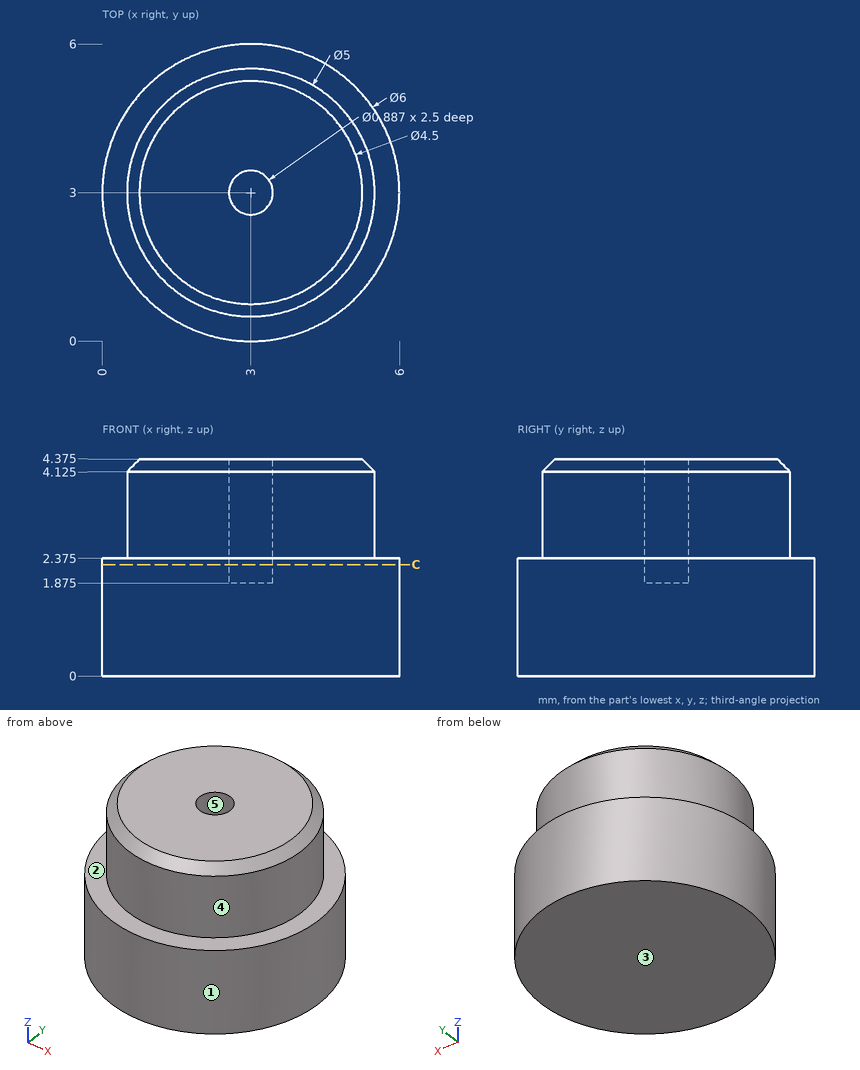
Could you check a few things on this drawing? It's one solid part, dimensions in mm from its lowest x, y, z. A direction names the side the tool comes from. Round coordinates to 2 decimals unless told otherwise and drop trailing zeros. Loops run counter-clockwise (first coordinate to the right, second up) from the corner with the lowest first, then second, coordinate; pieces in that order, holes last.
Q1. On a 3-axis mill with a long thin cutter (end or side, diameter ignored), from which of +Z, -Z, +X, -X, +Y, -Y can I reach the whole of each face in a straight line? I mean the marked faces 1 and 2. Say none if no direction works.
Q2. Thinking about a two-plate mould opening in X: for the marked faces 3, 4 and 5, which applies, pulls with the +X half, pulls with the -X half, needs draft (parallel to the pull), parting line crosses it, or undercut?
Q3. For P1, Ø1.5, axis at y = 2, z = 4, coming from the +X side; P2, Ø1, axis at y = 1, z = 1, coming from the +X side, each with a flat end and sliding along its axis, tell me the tip position at first contact or that it passes through.
Q4. I want a section at C-C (z = 2.25). Write out the boundary of the cut face in (x, y).
Q5. Please list where these lines run through material, in increasing order: L1, parallel to Y at x = 3, z = 3.35; L2, parallel to Z at x = 3.7, y = 5.6 (3 decimals); L3, parallel to Z at x = 5.05, y = 1.85.
Answer below:
1. face 1: +Z, -Z
1. face 2: +Z
2. face 3: needs draft
2. face 4: parting line crosses it
2. face 5: undercut
3. P1: stops at x = 5.49
3. P2: stops at x = 5.6
4. outline: circle Ø6 at (3, 3); hole circle Ø0.89 at (3, 3)
5. L1: y = 0.5 to 2.56, 3.44 to 5.5
5. L2: z = 0 to 2.375
5. L3: z = 0 to 4.27
